Part model, mm, in its own coordinate system. A direction names the side the tool comes from. Coordinates: 2 decimals unless noted, no trailing zeros. Loops run counter-clockwise (first coordinate to the right, second up) from the corner with the lowest first, then second, coordinate; pieces in that order, holes last.
Autodesk Inventor part; units mm, degrees
ref_plane "Work Plane1" through (0, 0, 8) normal (0, 0, -1) x (-1, 0, 0)
ref_plane "YZ Plane" through (0, 0, 0) normal (1, 0, 0) x (0, 1, 0)
ref_plane "XZ Plane" through (0, 0, 0) normal (0, 1, 0) x (-1, 0, 0)
sketch "Sketch1" plane through (0, 0, 0) normal (0, 0, 1) x (1, 0, 0)
  line L0 (-20, 10) -> (35, 10)
  line L1 (35, 10) -> (35, -10)
  line L2 (35, -10) -> (-20, -10)
  line L3 (-20, -10) -> (-20, 10)
  line L4 (-31, 0) -> (46, 0)
  line L5 (0, -14) -> (0, 14)
  point P0 (0, 0)
  point P1 (-10, 0)
  point P2 (10, 0)
  point P3 (27.5, 0)
  dimension "d0" = 20
  dimension "d2" = 55
  dimension "d8" = 20
  dimension "d9" = 20
  dimension "d10" = 7.5
extrude "Extrusion1" add sketch "Sketch1" along normal blind 16
sketch "Sketch2" plane through (0, 0, 0) normal (0, 0, 1) x (1, 0, 0)
  line L0 (-20, 10) -> (35, 10)
  line L1 (35, 10) -> (35, -10)
  line L2 (35, -10) -> (-20, -10)
  line L3 (-20, -10) -> (-20, 10)
  line L4 (0, 14) -> (0, -14)
  line L5 (-31, 0) -> (46, 0)
  point P0 (0, 0)
  point P1 (-10, 0)
  point P2 (10, 0)
  dimension "d38" = 20
  dimension "d39" = 55
  dimension "d41" = 20
hole "Hole4" at (-10, 0, 0) at (10, 0, 0) direction (0, 0, 1) diameter 4.2 end through all counterbore diameter 8.65 counterbore depth 12.8
sketch "Sketch3" plane through (0, 0, 0) normal (0, 0, 1) x (1, 0, 0)
  line L0 (-20, 10) -> (35, 10)
  line L1 (35, 10) -> (35, -10)
  line L2 (35, -10) -> (-20, -10)
  line L3 (-20, -10) -> (-20, 10)
  point P0 (0, 0)
  point P1 (-10, 0)
  point P2 (10, 0)
  point P3 (27.5, 0)
  dimension "d50" = 20
  dimension "d51" = 55
  dimension "d52" = 20
  dimension "d53" = 7.5
hole "Hole5" at (27.5, 0, 0) direction (0, 0, 1) diameter 4.2 depth 8 tip angle 118 counterbore diameter 8.65 counterbore depth 3.2
ref_plane "Work Plane1" through (0, 0, 8) normal (0, 0, -1) x (-1, 0, 0)
sketch "Sketch5" plane through (0, 0, 8) normal (0, 0, -1) x (-1, 0, 0)
  line L0 (-40, -10) -> (0, -10)
  line L1 (0, -10) -> (0, 10)
  line L2 (0, 10) -> (-40, 10)
  line L3 (-40, 10) -> (-40, -10)
  line L4 (49, 0) -> (-49, 0)
  line L5 (0, -14) -> (0, 14)
  point P0 (0, 0)
  point P1 (0, 0)
  dimension "d64" = 20
  dimension "d65" = 40
extrude "Extrusion2" cut sketch "Sketch5" along normal mid plane 1
sketch "Sketch6" plane through (0, 0, 0) normal (0, 1, 0) x (-1, 0, 0)
  line L0 (0, 7.5) -> (0, 8.5)
  circle A0 centre (0, 8) radius 4.6
  point P0 (0, 0)
  dimension "d68" = 9.2
extrude "Extrusion3" cut sketch "Sketch6" along normal mid plane 20
hole "Hole6" at (27.5, 0, 0) direction (0, 0, 1) diameter 3.3 end through all
properties part number "Lezerlefogov3"
Q1. Tool access for faces 1 (the cylindrical face through (6.353, 2.325, 10.68)), 2 (the flat face through (20, 0, 8.5)), 3 (the flat face through (35, 0, 12)): list every direction of +Z, -Z, +X, -X, +Y, -Y with a clear straight run to the whole face (end or side of a thin tool).
Q2. Saw through at A-A (x = 10). List the corners of the cut face in (y, z) (3 decimals), plus the area to 3 significant figures.
Q3. Probe line 1 (X direction, y = 0, z = 14.6); line 2 (Y direction, x = 10, z = 5) (3 decimals); line 3 (Z direction, x = 20, y = -7.5). List the from-to ranges inside material, lowest first.
Q4. Mould opens along Y. For faces 4 (the flat face through (8, -10, 6)), 5 (the flat face through (7, 0, 16)), 6 (the cylindrical face through (25.73, 1.13, 5.38)), 7 (the flat face through (7, 10, 10)) say: released by +Y, released by -Y, zero draft, split by the parting line, or undercut.
Q5. Drop flat-ended pins along their axis: P1, Ø4.5, axis at x = 27.5, y = 0, coming from the -Z side; P2, Ø3.5, axis at x = 10, y = 0, coming from the +Z side; P3, Ø5, axis at x = -10, y = 0, coming from the -Z side. Give the stop position or say it passes through.
Q6. Saw through at C-C (x = 0). List the corners of the cut face in (y, z), plus the area to 3 significant figures.
Q7. Saw through at D-D (z = 1.75). List the corners of the cut face in (x, y) (3 decimals), plus the area to 3 significant figures.
Q8. Saw through at B-B (z = 11.5). List the corners of the cut face in (x, y) (3 decimals), plus the area to 3 significant figures.
Checked values:
1. face 1: -Z
1. face 2: +X, +Y, -Y
1. face 3: +Z, -Z, +X, +Y, -Y
2. outline: (-10, 0) - (-4.325, 0) - (-4.325, 7.5) - (-10, 7.5) - close; (-10, 8.5) - (-4.325, 8.5) - (-4.325, 12.8) - (-2.1, 12.8) - (-2.1, 16) - (-10, 16) - close; (2.1, 12.8) - (4.325, 12.8) - (4.325, 8.5) - (10, 8.5) - (10, 16) - (2.1, 16) - close; (4.325, 0) - (10, 0) - (10, 7.5) - (4.325, 7.5) - close
2. area: 184 mm2
3. line 1: x = -20 to -12.1, -7.9 to 7.9, 12.1 to 25.85, 29.15 to 35
3. line 2: y = -10 to -4.325, 4.325 to 10
3. line 3: z = 0 to 7.5, 8.5 to 16
4. face 4: released by -Y
4. face 5: zero draft
4. face 6: undercut
4. face 7: released by +Y
5. P1: stops at z = 3.2
5. P2: passes through
5. P3: stops at z = 12.8
6. outline: (-10, 0) - (10, 0) - (10, 3.4) - (-10, 3.4) - close; (-10, 12.6) - (10, 12.6) - (10, 16) - (-10, 16) - close
6. area: 136 mm2
7. outline: (-20, -10) - (35, -10) - (35, 10) - (-20, 10) - close; hole circle Ø8.65 at (-10, 0); hole circle Ø8.65 at (10, 0); hole circle Ø8.65 at (27.5, 0)
7. area: 924 mm2
8. outline: (-20, -10) - (-2.985, -10) - (-2.985, 10) - (-20, 10) - close; (2.985, -10) - (35, -10) - (35, 10) - (2.985, 10) - close; hole circle Ø8.65 at (-10, 0); hole circle Ø8.65 at (10, 0); hole circle Ø3.3 at (27.5, 0)
8. area: 855 mm2
